```python
from build123d import *

# Parameters (mm, degrees)
F1_DEPTH = 7
F2_R     = 2.54


# Not quite as in the source:
# - a feature names something its author has since deleted; it is built from what else it names


with BuildPart() as f1:
    # F0 (on Top) → F1 (new body)
    with BuildSketch(Plane.XY):
        with BuildLine():
            ThreePointArc((12.7, 33.0220452561), (-20.3035705189, 26.2868814104), (-17.6006612279, -7.2882936508))
            ThreePointArc((-17.6006612279, -7.2882936508), (-8.6968003579, -16.9489870947), (4.3435297347, -18.5482141848))
            ThreePointArc((4.3435297347, -18.5482141848), (-11.7341390993, -24.436637764), (-26.0457140188, -15.0375))
            Line((-26.0457140188, -15.0375), (-34.9479300767, -5.5125))
            ThreePointArc((-34.9479300767, -5.5125), (-12.6133218282, -30.7268485621), (15.1121780658, -11.5984729214))
            ThreePointArc((15.1121780658, -11.5984729214), (19.0266535713, 0.9428435058), (13.8914598115, 13.0357141848))
            ThreePointArc((13.8914598115, 13.0357141848), (27.0298186363, 2.0562563305), (26.0457140188, -15.0375))
            Line((26.0457140188, -15.0375), (22.2479300767, -27.5095452561))
            ThreePointArc((22.2479300767, -27.5095452561), (32.9168923471, 4.4399671517), (2.4884831621, 18.8867665722))
            ThreePointArc((2.4884831621, 18.8867665722), (-10.3298532135, 16.0061435889), (-18.2349895462, 5.5125))
            ThreePointArc((-18.2349895462, 5.5125), (-15.295679537, 22.3803814335), (0, 30.075))
            Line((0, 30.075), (12.7, 33.0220452561))
        make_face()
        with BuildLine():
            ThreePointArc((0.0913914699, 11.0246211998), (7.8280973408, 7.7634732577), (11.025, 0))
            ThreePointArc((11.025, 0), (10.6610677893, -2.8093163923), (9.5932977611, -5.4331632653))
            ThreePointArc((9.5932977611, -5.4331632653), (9.5479300767, -5.5125), (9.5019062912, -5.5914579345))
            ThreePointArc((9.5019062912, -5.5914579345), (0, -11.025), (-9.5019062912, -5.5914579345))
            ThreePointArc((-9.5019062912, -5.5914579345), (-9.5479300767, -5.5125), (-9.5932977611, -5.4331632653))
            ThreePointArc((-9.5932977611, -5.4331632653), (-9.5479300767, 5.5125), (-0.0913914699, 11.0246211998))
            ThreePointArc((-0.0913914699, 11.0246211998), (0, 11.025), (0.0913914699, 11.0246211998))
        make_face(mode=Mode.SUBTRACT)
    extrude(amount=F1_DEPTH)

    # F2
    f2_edges = [f1.edges().sort_by_distance(p)[0] for p in [
        (12.7, 33.022045, 3.5),
        (22.24793, -27.509545, 3.5),
        (-34.94793, -5.5125, 3.5),
    ]]
    fillet(f2_edges, radius=F2_R)


solid = f1.part
```
Geometry check sheet. Reference: the model listing, model coordinates, mm. A direction names the side the tool comes from. Give positions to 0.01 mm unless a question says otherwise; leave off trailing zeros. Write each loop counter-clockwise with the first axis right and the second up, starting at its lowest first coordinate (ties: lowest second). Pieces come first, ordered by that corner, then holes. Notation, with made-up numbers: (31, 13.5) -> (64, 13.5) arc R29 ccw to (64, 42.5) -> close; hole circle Ø5 at (-14.5, -5). An arc over 180 degrees is marked (long way). Use one line per item in the form item = value.
Item 1: Depth check by flat-ended pin: pin 1 Ø4 at (x, z) = (-2.5, 1) entering from -Y; pin 2 Ø2 at (y, z) = (19, 6) entering from +X. Enter the tip coordinate at first touch or a pass-through.
Results list:
pin_1 = -30.41
pin_2 = 19.16
Item 2: Access from +Z, -Z, +X, -X, +Y, -Y to the whole of each face (thin tool, end or side, straight path). Record for faces 4 (the flat face through (-27.56, -13.42, 3.45)), 5 (the flat face through (25.4, -17.16, 3.45)), 6 (the flat face through (2.16, 30.576, 3.451)).
Results list:
face_4 = +Z, -Z, +Y
face_5 = +Z, -Z
face_6 = +Z, -Z, +X
Item 3: Sectioned sample at D-D on x = -23.5. Enter the section's corners in (y, z), plus the area to 3 significant figures.
Results list:
outline = (-26.74, 0) -> (-18.48, 0) -> (-18.48, 7) -> (-26.74, 7) -> close; (1.39, 0) -> (20.66, 0) -> (20.66, 7) -> (1.39, 7) -> close
area = 193 mm2
Item 4: Mould release check, pull along Y, two halves, no side actions. Record for faces 1 (the flat face through (0, -12, 7)), 2 (the cylindrical face through (-8.548, -30.893, 3.451)), 3 (the cylindrical face through (26.93, 2.28, 3.45)): released by +Y, released by -Y, zero draft, split by the parting line, or undercut.
Results list:
face_1 = zero draft
face_2 = released by -Y
face_3 = undercut
Item 5: Sectioned sample at B-B on x = -12.5. Enter the section's corners in (y, z), plus the area to 3 significant figures.
Results list:
outline = (-30.74, 0) -> (-24.33, 0) -> (-24.33, 7) -> (-30.74, 7) -> close; (-14.38, 0) -> (14.38, 0) -> (14.38, 7) -> (-14.38, 7) -> close; (25.4, 0) -> (33.14, 0) -> (33.14, 7) -> (25.4, 7) -> close
area = 300 mm2
Item 6: Scan lines: line 1 (Y direction, x = -11.5, z = 3.5); line 2 (Y direction, x = -9.5, z = 0.5); line 3 (X direction, y = -2.5, z = 1). Record each from-to range of solid material in increasing order.
Results list:
line_1 = -30.84 to -24.46, -15.19 to 15.19, 26.21 to 33.67
line_2 = -30.91 to -24.56, -16.51 to -5.59, 5.59 to 16.51, 27.54 to 34.58
line_3 = -21.5 to -10.74, 10.74 to 18.89, 28.36 to 34.77
Item 7: Sectioned sample at A-A on y = 12. Enter the section's corners in (x, z), plus the area to 3 significant figures.
Results list:
outline = (-25.38, 0) -> (-19.03, 0) -> (-19.03, 7) -> (-25.38, 7) -> close; (-14.8, 0) -> (14.8, 0) -> (14.8, 7) -> (-14.8, 7) -> close; (17.05, 0) -> (27.95, 0) -> (27.95, 7) -> (17.05, 7) -> close
area = 328 mm2
